from build123d import *

# Parameters (mm, degrees)
FILLET1_R                        = 10
M10X1_0_TAPPED_HOLE1_D           = 9
M10X1_0_TAPPED_HOLE1_DEPTH       = 25
M10X1_0_TAPPED_HOLE1_CSINK_D     = 10.5
M10X1_0_TAPPED_HOLE1_CSINK_ANGLE = 90
M10X1_0_TAPPED_HOLE1_TIP         = 2.703872786


with BuildPart() as part:
    # Sketch1 → Revolve1 (revolve)
    with BuildSketch(Plane.XY):
        with BuildLine():
            Line((-20, 0), (35, 0))
            Line((35, 0), (35, 9))
            Line((35, 9), (17.860571099, 9))
            ThreePointArc((17.860571099, 9), (-4.625396092, 19.457793066), (-20, 0))
        make_face()
    revolve(axis=Axis((0, 0, 0), (1, 0, 0)))

    # Fillet1
    fillet1_edges = [part.edges().sort_by_distance(p)[0] for p in [
        (17.860571099, -9, 0),
    ]]
    fillet(fillet1_edges, radius=FILLET1_R)

    # M10x1.0 Tapped Hole1
    with Locations(Plane(origin=(35, 0, 0), x_dir=(0, 0, -1), z_dir=(1, 0, 0))):
        with Locations((0, 0)):
            CounterSinkHole(M10X1_0_TAPPED_HOLE1_D / 2, M10X1_0_TAPPED_HOLE1_CSINK_D / 2, depth=M10X1_0_TAPPED_HOLE1_DEPTH, counter_sink_angle=M10X1_0_TAPPED_HOLE1_CSINK_ANGLE)
            with Locations((0, 0, -(M10X1_0_TAPPED_HOLE1_DEPTH + M10X1_0_TAPPED_HOLE1_TIP / 2))):  # 118° drill point
                Cone(0, M10X1_0_TAPPED_HOLE1_D / 2, M10X1_0_TAPPED_HOLE1_TIP, mode=Mode.SUBTRACT)


solid = part.part
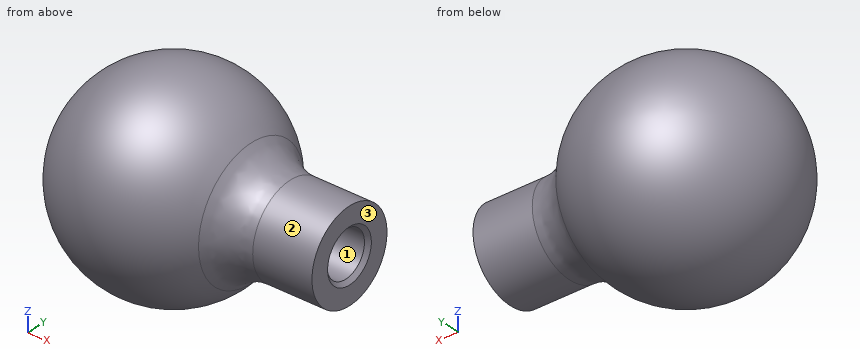
The listing builds one solid part. Answer for the finished solid, in the listing's coordinates (mm). Face numbers are marked on the shaded views. Coordinates: 2 decimals unless noted, no trailing zeros. Write each loop counter-clockwise with the first axis right and the second up, starting at its lowest first coordinate (ties: lowest second). Pieces come first, ordered by that corner, then holes. Notation, with made-up numbers: (16, -7.75) -> (57, -7.75) arc R28 ccw to (57, 12.25) -> close; hole circle Ø10 at (42.25, -20). An arc over 180 degrees is marked (long way). One line per question, with ' | ' between items.
1. Section A-A (x = 32.5) is taken. Determine the outline of the cut face in (y, z), and give its area (3 significant figures).
Verdict:
outline: circle Ø18 at (0, 0); hole circle Ø9 at (0, 0) | area: 191 mm^2
2. Straight lines are drawn through the part: line 1 (Y direction, x = 24, z = 0); line 2 (Z direction, x = 16.75, y = 0). For each, find the intervals that lie inside material, in ascending order.
Verdict:
line 1: y = -9 to -4.5, 4.5 to 9 | line 2: z = -11.37 to -4.5, 4.5 to 11.37
3. Section B-B (x = -1) is taken. Determine the outline of the cut face in (y, z), and give its area (3 significant figures).
Verdict:
outline: circle Ø39.95 at (0, 0) | area: 1,250 mm^2
4. For a pull along Y with two mould halves and no side action, classify the marked faces 1, 2 and 3 as released by +Y, released by -Y, zero draft, split by the parting line, or undercut.
Verdict:
face 1: undercut | face 2: split by the parting line | face 3: zero draft
5. Given pin 1 Ø12 at (y, z) = (-7, -14) entering from -X; pin 2 Ø12 at (x, z) = (10.5, -4.5) entering from +Y; pin 3 Ø5 at (y, z) = (-9.5, -8) entering from -X, each flat-ended and moving along its own axis, determine where each tip first touches the part or whether it passes through.
Verdict:
pin 1: stops at x = -17.52 | pin 2: stops at y = 19.25 | pin 3: stops at x = -17.37
6. Section C-C (z = 14.5) is taken. Determine the outline of the cut face in (x, y).
Verdict:
outline: circle Ø27.55 at (0, 0)
